Autodesk Inventor part; units mm, degrees
ref_plane "Arbeitsebene1" through (0, 2, 0) normal (0, 1, 0) x (-1, 0, 0)
ref_plane "YZ Plane" through (0, 0, 0) normal (1, 0, 0) x (0, 1, 0)
ref_plane "XY Plane" through (0, 0, 0) normal (0, 0, 1) x (1, 0, 0)
sketch "Skizze1" plane through (0, 0, 0) normal (0, 1, 0) x (-1, 0, 0)
  line L0 (-5, 5) -> (5, 5)
  line L1 (5, 5) -> (5, -5)
  line L2 (5, -5) -> (-5, -5)
  line L3 (-5, -5) -> (-5, 5)
  line L4 (-5, 5) -> (5, -5) construction
  line L5 (5, 5) -> (-5, -5) construction
  point P0 (0, 0)
  dimension "d0" = 10
  dimension "d1" = 10
extrude "Extrusion1" add sketch "Skizze1" along normal mid plane 5.5
sketch "Skizze2" plane through (5, -2.75, -5) normal (1, 0, 0) x (0, 0, -1)
  circle A0 centre (-5, 2.75) radius 2.5
  dimension "d4" = 5
extrude "Extrusion2" add sketch "Skizze2" along normal blind 6.5
sketch "Skizze3" plane through (11.5, 0, 0) normal (1, 0, 0) x (0, 0, -1)
  circle A0 centre (0, 0) radius 2.5
  circle A1 centre (0, 0) radius 2
  dimension "d7" = 4
extrude "Extrusion3" add sketch "Skizze3" along normal blind 74 contours A1
sketch "Skizze4" plane through (0, 2.75, 0) normal (0, 1, 0) x (1, 0, 0)
  point P0 (0, 0)
  point P1 (0, 0)
hole "Bohrung1" at (0, 2.75, 0) direction (0, -1, 0) diameter 5.5 depth 5.5
ref_plane "Arbeitsebene1" through (0, 2, 0) normal (0, 1, 0) x (-1, 0, 0)
sketch "Skizze5" plane through (0, 2, 0) normal (0, 1, 0) x (-1, 0, 0)
  line L0 (-85.5, 2) -> (-85.5, -2)
  point P0 (0, 0)
  point P1 (-83, 0)
  dimension "d18" = 2.5
hole "Bohrung2" at (83, 2, 0) direction (0, -1, 0) diameter 2 end through all
chamfer "Fasen1" distance 1 angle 45 1 edges at (85.5, 0, 2)
properties part number "BMS_24" material "Titan"
Design review of the part built by this model. Coordinates are the model's own, in mm. A direction names the side the tool comes from. Give positions to 0.01 mm unless a question says otherwise; leave off trailing zeros. Loops run counter-clockwise (first coordinate to the right, second up) from the corner with the lowest first, then second, coordinate; pieces in that order, holes last. Notation, with made-up numbers: (69.25, -8.5) -> (120.25, -8.5) arc R22 cw to (120.25, 10.5) -> close; hole circle Ø7 at (44.25, 64.5). An arc over 180 degrees is marked (long way). One line per question, with ' | ' between items. Start each with the question number.
(1) We need section B-B (z = 0). State the section outline as (x, y) points, and give its area (3 significant figures).
(2) For line 1 (X direction, y = -0.8, z = 0); line 2 (X direction, y = 1.2, z = 3.25); line 3 (Y direction, x = 74, z = -0.25), list the stretches that pass through material, from the lowest coordinate up.
(3) We need section C-C (z = -3.75). State the section outline as (x, y) points, and give its area (3 significant figures).
(4) We need section D-D (x = 41). State the section outline as (y, z) points.
(5) Insertion check: P1, Ø1, axis at x = 45.5, y = -2, coming from the -Z side; P2, Ø1, axis at x = 43, z = 2, coming from the +Y side; P3, Ø4, axis at x = 43, z = -1, coming from the +Y side. Each pin has a flat end and moves straight along its axis. Give the tip position at first contact, or say it passes through.
(6) We need section A-A (x = 0). State the section outline as (y, z) points.
(7) Draft analysis for pull direction Z (two halves, no side actions). For faces 1 (the face through (0, 0, 5)), 2 (the face through (83, 0, 1)), 3 (the face through (0, 0, -5)), 4 (the face through (2.685, -0.038, -0.596)), state which applies: +Z half, -Z half, draft (parallel to the pull), parting line (faces both ways), or undercut.
(8) For faces 5 (the face through (5, 2.4, -1.2)), 6 (the face through (-5, 0, 0)), list the 3-axis set-ups (+Z, -Z, +X, -X, +Y, -Y) from which the entire face can be reached by the end or side of a thin tool; tool diameter is ignored.
The answers:
1) outline: (-5, -2.75) -> (-2.75, -2.75) -> (-2.75, 2.75) -> (-5, 2.75) -> close; (2.75, -2.75) -> (5, -2.75) -> (5, -2.5) -> (11.5, -2.5) -> (11.5, -2) -> (82, -2) -> (82, 2) -> (11.5, 2) -> (11.5, 2.5) -> (5, 2.5) -> (5, 2.75) -> (2.75, 2.75) -> close; (84, -2) -> (84.5, -2) -> (85.5, -1) -> (85.5, 1) -> (84.5, 2) -> (84, 2) -> close | area: 344 mm^2
2) line 1: x = -5 to -2.75, 2.75 to 82, 84 to 85.5 | line 2: x = -5 to 5 | line 3: y = -1.98 to 1.98
3) outline: (-5, -2.75) -> (5, -2.75) -> (5, 2.75) -> (-5, 2.75) -> close | area: 55.0 mm^2
4) outline: circle Ø4 at (0, 0)
5) P1: stops at z = -1.32 | P2: stops at y = 1.32 | P3: stops at y = 2
6) outline: (-2.75, -5) -> (2.75, -5) -> (2.75, -2.75) -> (-2.75, -2.75) -> close; (-2.75, 2.75) -> (2.75, 2.75) -> (2.75, 5) -> (-2.75, 5) -> close
7) face 1: +Z half | face 2: undercut | face 3: -Z half | face 4: undercut
8) face 5: +X | face 6: +Z, -Z, -X, +Y, -Y
